Geometry: final body of the model. Coordinates: model frame, mm. A direction names the side the tool comes from. Round coordinates to 2 decimals unless told otherwise and drop trailing zeros. Loops run counter-clockwise (first coordinate to the right, second up) from the corner with the lowest first, then second, coordinate; pieces in that order, holes last. Notation, with made-up numbers: M -18,81.5 L 21,81.5 A15 cw 21,93.5 Z; hole C 37,85 d6. An arc over 180 degrees is marked long. Return JSON: item names as keys, results as strings.
from build123d import *

# Parameters (mm, degrees)
SKETCH1_R           = 1.5
SKETCH1_R_2         = 1.75
BOSS_EXTRUDE1_DEPTH = 2.5
CHAMFER1_SIZE       = 1
CUT_EXTRUDE1_REACH  = 35.077
SKETCH2_W           = 8
SKETCH2_H           = 24
FILLET1_R           = 2
SKETCH3_W           = 4.5
SKETCH3_H           = 59
CUT_EXTRUDE2_DEPTH  = 1.25


with BuildPart() as part:
    # Sketch1 → Boss-Extrude1 (new body)
    with BuildSketch(Plane(origin=(0, 0, 0), x_dir=(1, 0, 0), z_dir=(0, 1, 0))):
        with BuildLine():
            Line((11.125, 29.5), (-11.125, 29.5))
            ThreePointArc((-11.125, 29.5), (-14.714662754, 25.370077916), (-10.125, 22.390660034))
            Line((-10.125, 22.390660034), (-10.125, -22.390660034))
            ThreePointArc((-10.125, -22.390660034), (-14.714662754, -25.370077916), (-11.125, -29.5))
            Line((-11.125, -29.5), (11.125, -29.5))
            ThreePointArc((11.125, -29.5), (14.714662754, -25.370077916), (10.125, -22.390660034))
            Line((10.125, -22.390660034), (10.125, 22.390660034))
            ThreePointArc((10.125, 22.390660034), (14.714662754, 25.370077916), (11.125, 29.5))
        make_face()
        with Locations(Location((-6.5, 7.875, 0), (0, 0, 270))):
            Circle(SKETCH1_R, mode=Mode.SUBTRACT)
        with Locations(Location((6.5, 20.375, 0), (0, 0, 270))):
            Circle(SKETCH1_R, mode=Mode.SUBTRACT)
        with Locations(Location((-6.5, 20.375, 0), (0, 0, 270))):
            Circle(SKETCH1_R, mode=Mode.SUBTRACT)
        with Locations(Location((6.5, 7.875, 0), (0, 0, 270))):
            Circle(SKETCH1_R, mode=Mode.SUBTRACT)
        with Locations(Location((-11.125, 25.875, 0), (0, 0, 270))):
            Circle(SKETCH1_R_2, mode=Mode.SUBTRACT)
        with Locations(Location((11.125, 25.875, 0), (0, 0, 270))):
            Circle(SKETCH1_R_2, mode=Mode.SUBTRACT)
        with Locations(Location((-11.125, -25.875, 0), (0, 0, 270))):
            Circle(SKETCH1_R_2, mode=Mode.SUBTRACT)
        with Locations(Location((11.125, -25.875, 0), (0, 0, 270))):
            Circle(SKETCH1_R_2, mode=Mode.SUBTRACT)
    extrude(amount=BOSS_EXTRUDE1_DEPTH)

    # Chamfer1
    chamfer1_edges = [part.edges().sort_by_distance(p)[0] for p in [
        (6.5, 2.5, -21.875),
        (-6.5, 2.5, -21.875),
        (-6.5, 2.5, -9.375),
        (6.5, 2.5, -9.375),
    ]]
    chamfer(chamfer1_edges, length=CHAMFER1_SIZE)

    # Sketch2 → Cut-Extrude1 (cut, up to next)
    with BuildSketch(Plane(origin=(0, 2.5, 0), x_dir=(1, 0, 0), z_dir=(0, 1, 0)), mode=Mode.PRIVATE) as cut_extrude1_sk1:
        with Locations((0, -11.5)):
            Rectangle(SKETCH2_W, SKETCH2_H)
    cut_extrude1_tool1 = extrude(cut_extrude1_sk1.sketch, amount=-CUT_EXTRUDE1_REACH, mode=Mode.PRIVATE) & part.part
    add(cut_extrude1_tool1.solids().sort_by_distance((0, 2.5, 11.5))[0], mode=Mode.SUBTRACT)

    # Fillet1
    fillet1_edges = [part.edges().sort_by_distance(p)[0] for p in [
        (-10.125, 1.25, 22.390660034),
        (-10.125, 1.25, -22.390660034),
        (10.125, 1.25, -22.390660034),
        (10.125, 1.25, 22.390660034),
        (4, 1.25, -0.5),
        (4, 1.25, 23.5),
        (-4, 1.25, 23.5),
        (-4, 1.25, -0.5),
    ]]
    fillet(fillet1_edges, radius=FILLET1_R)

    # Sketch3 → Cut-Extrude2 (cut)
    with BuildSketch(Plane.XZ):
        Rectangle(SKETCH3_W, SKETCH3_H)
    extrude(amount=-CUT_EXTRUDE2_DEPTH, mode=Mode.SUBTRACT)


solid = part.part
Q1. Pin query (flat end, axial travel): pin 1 (1.5 mm diameter, centred on y = 2, z = -2, fed in from +X) (3 decimals); pin 2 (1.5 mm diameter, centred on x = -6, z = -22, fed in from +Y); pin 3 (0.6 mm diameter, centred on y = 1, z = 25, fed in from +X); pin 4 (3.5 mm diameter, centred on x = -6.5, z = -20.375, fed in from -Y). Return the tip coordinate at first contact, or that it passes through.
Determined:
{"pin 1": "stops at x = 10.125", "pin 2": "stops at y = 2.45", "pin 3": "stops at x = 14.7", "pin 4": "stops at y = 0"}
Q2. Section query C-C (x = 1). Output: boundary loops of the cut face in (y, z).
Determined:
{"outline": "M 1.25,-29.5 L 2.5,-29.5 L 2.5,-0.5 L 1.25,-0.5 Z; M 1.25,23.5 L 2.5,23.5 L 2.5,29.5 L 1.25,29.5 Z"}
Q3. Material intervals for L1, parallel to X at y = 2.4, z = 26; L2, parallel to X at y = 0.3, z = -26; L3, parallel to X at y = 0.35, z = 1.5 (3 decimals), sorted ascending.
Determined:
{"L1": "x = -14.75 to -12.87, -9.38 to 9.38, 12.87 to 14.75", "L2": "x = -14.75 to -12.87, -9.38 to -2.25, 2.25 to 9.38, 12.87 to 14.75", "L3": "x = -10.125 to -4, 4 to 10.125"}
Q4. Section query B-B (x = -6.5). Output: boundary loops of the cut face in (y, z) (3 decimals).
Determined:
{"outline": "M 0,-29.5 L 2.5,-29.5 L 2.5,-22.875 L 1.5,-21.875 L 0,-21.875 Z; M 0,-18.875 L 1.5,-18.875 L 2.5,-17.875 L 2.5,-10.375 L 1.5,-9.375 L 0,-9.375 Z; M 0,-6.375 L 1.5,-6.375 L 2.5,-5.375 L 2.5,29.5 L 0,29.5 Z"}
Q5. Pull-direction query (Z, two-part tool) for faces 1 (the cylindrical face through (-10.58, 1.27, 21.61)), 2 (the flat face through (2.25, 1, 26)), 3 (the flat face through (0, 2, -29.5)); classes: pulls with the +Z half, pulls with the -Z half, needs draft (parallel to the pull), parting line crosses it, or undercut.
Determined:
{"face 1": "undercut", "face 2": "needs draft", "face 3": "pulls with the -Z half"}
Q6. Section query D-D (z = -25). Output: boundary loops of the cut face in (x, y).
Determined:
{"outline": "M -14.64,0 L -12.64,0 L -12.64,2.5 L -14.64,2.5 Z; M -9.61,0 L -2.25,0 L -2.25,1.25 L 2.25,1.25 L 2.25,0 L 9.61,0 L 9.61,2.5 L -9.61,2.5 Z; M 12.64,0 L 14.64,0 L 14.64,2.5 L 12.64,2.5 Z"}
Q7. Reachability of faces 4 (the cylindrical face through (-10.603, 1.268, -21.637)), 5 (the cylindrical face through (10.603, 1.268, -21.637)), 6 (the flat face through (-2.25, 1, 26)) from +Z, -Z, +X, -X, +Y, -Y: full face, straight path, thin tool, end or side. Return the list, or none.
Determined:
{"face 4": "-X, +Y, -Y", "face 5": "+X, +Y, -Y", "face 6": "+Z, -Z, -Y"}
Q8. Section query A-A (z = 11). Output: boundary loops of the cut face in (x, y) (3 decimals), plus the area to 3 significant figures.
Determined:
{"outline": "M -10.125,0 L -4,0 L -4,2.5 L -10.125,2.5 Z; M 4,0 L 10.125,0 L 10.125,2.5 L 4,2.5 Z", "area": "30.6 mm^2"}
